Geometry: final body of the model. Coordinates: model frame, mm. A direction names the side the tool comes from. Coordinates: 2 decimals unless noted, no trailing zeros. Order: outer loops, then holes, each group sorted by start corner. A loop starts at its lowest first (then second) coordinate and runs counter-clockwise, first axis right, second up. Notation, with made-up numbers: (33, 87) -> (51, 87) arc R11 cw to (51, 105) -> close; hole circle Ø5 at (73, 64.25). An arc over 180 degrees is marked (long way). Answer in a Markdown table with one row per item. Add a question column.
1) Section query B-B on x = 57.25. Return the cut outline in (y, z).
2) Ray query, line 1 (X direction, y = 0.85, z = -37.25); line 2 (Z direction, x = 46, y = 6.5); line 3 (Y direction, x = 34, z = -15.5). Return the intervals inside material, ascending. Write a range as from..to.
3) Set-up query: faces 5 (the face through (41, 13, -16)), 6 (the face through (20.436, 10, -19)), 7 (the face through (57, 9, -32)). Return all of +Z, -Z, +X, -X, +Y, -Y with unobstructed straight access to the full face (end or side cutting, diameter ignored); none if empty.
4) Contact query for flat-ended pins moving along their axis: P1, Ø2, axis at x = 15.5, z = -25.5, coming from the +Y side; P2, Ø2, axis at y = 6, z = -18, coming from the +X side; P3, Ø8.5, axis at x = 12.5, y = 13, coming from the -Z side. Output: stop coordinate, or through.
5) Section query D-D on x = 13. Return the cut outline in (y, z), then the cut area to 3 significant figures.
6) Pull-direction query (X, two-part tool) for faces 1 (the face through (51, 7, -9.117)), 2 (the face through (2.21, 0.51, -35.96)), 3 (the face through (61.554, 5, -32)), 4 (the face through (52.647, 5, -32)); classes: +X half, -X half, draft (parallel to the pull), parting line (faces both ways), or undercut.
7) Section query A-A on z = -37.25. Return the cut outline in (x, y).
8) Section query C-C on y = 5. Return the cut outline in (x, z), then the cut area to 3 significant figures.
```python
from build123d import *

# Parameters (mm, degrees)
SKETCH1_W           = 60
SKETCH1_H           = 40
BOSS_EXTRUDE1_DEPTH = 1
SKETCH2_R           = 1.4
CUT_EXTRUDE1_DEPTH  = 73.117958928
SKETCH3_R           = 1.794713796
SKETCH3_W           = 11.029321298
SKETCH3_H           = 9.406259618
BOSS_EXTRUDE2_DEPTH = 12
SKETCH4_W           = 8.907146541
SKETCH4_H           = 4.90887134
BOSS_EXTRUDE3_DEPTH = 8
SKETCH5_W           = 7.89622208
SKETCH5_H           = 4.078620146
SKETCH5_W_2         = 8.030698063
BOSS_EXTRUDE4_DEPTH = 18


with BuildPart() as part:
    # Sketch1 → Boss-Extrude1 (new body)
    with BuildSketch(Plane(origin=(0, 0, 0), x_dir=(1, 0, 0), z_dir=(0, 1, 0))):
        with Locations((30, 20)):
            Rectangle(SKETCH1_W, SKETCH1_H)
    extrude(amount=BOSS_EXTRUDE1_DEPTH)

    # Sketch2 → Cut-Extrude1 (cut, through all)
    with BuildSketch(Plane(origin=(0, 1, 0), x_dir=(1, 0, 0), z_dir=(0, 1, 0))):
        with Locations(Location((2.75, 37.25, 0), (0, 0, 270))):
            Circle(SKETCH2_R)
        with Locations(Location((57.25, 37.25, 0), (0, 0, 270))):
            Circle(SKETCH2_R)
        with Locations(Location((57.25, 2.75, 0), (0, 0, 270))):
            Circle(SKETCH2_R)
        with Locations(Location((2.75, 2.75, 0), (0, 0, 270))):
            Circle(SKETCH2_R)
    extrude(amount=-CUT_EXTRUDE1_DEPTH, mode=Mode.SUBTRACT)

    # Sketch3 → Boss-Extrude2 (add)
    with BuildSketch(Plane(origin=(0, 1, 0), x_dir=(1, 0, 0), z_dir=(0, 1, 0))):
        with Locations(Location((41.01670641, 16.304679201, 0), (0, 0, 90))):
            Circle(SKETCH3_R)
        with Locations((50.861034001, 13.82058061)):
            Rectangle(SKETCH3_W, SKETCH3_H)
    extrude(amount=BOSS_EXTRUDE2_DEPTH)

    # Sketch4 → Boss-Extrude3 (add)
    with BuildSketch(Plane(origin=(0, 1, 0), x_dir=(1, 0, 0), z_dir=(0, 1, 0))):
        with Locations((57.100404147, 31.839794384)):
            Rectangle(SKETCH4_W, SKETCH4_H)
    extrude(amount=BOSS_EXTRUDE3_DEPTH)

    # Sketch5 → Boss-Extrude4 (add)
    with BuildSketch(Plane(origin=(0, 1, 0), x_dir=(1, 0, 0), z_dir=(0, 1, 0))):
        with Locations((13.964882377, 18.540826958)):
            Rectangle(SKETCH5_W, SKETCH5_H)
        with Locations((24.451181127, 18.540826958)):
            Rectangle(SKETCH5_W_2, SKETCH5_H)
    extrude(amount=BOSS_EXTRUDE4_DEPTH)


solid = part.part
```
Result:
| question | item | result |
|---|---|---|
| 1 | outline | (0, -40) -> (1, -40) -> (1, -38.65) -> (0, -38.65) -> close; (0, -35.85) -> (1, -35.85) -> (1, -34.29) -> (9, -34.29) -> (9, -29.39) -> (1, -29.39) -> (1, -4.15) -> (0, -4.15) -> close; (0, -1.35) -> (1, -1.35) -> (1, 0) -> (0, 0) -> close |
| 2 | line 1 | 0..1.35, 4.15..55.85, 58.65..60 |
| 2 | line 2 | -18.52..-9.12 |
| 2 | line 3 | 0..1 |
| 3 | face 5 | +Z, -Z, +X, +Y |
| 3 | face 6 | +Z, -Z, +Y |
| 3 | face 7 | -Z, +X, -X, +Y |
| 4 | P1 | y = 1 |
| 4 | P2 | x = 56.38 |
| 4 | P3 | z = -20.58 |
| 5 | outline | (0, -40) -> (1, -40) -> (1, -20.58) -> (19, -20.58) -> (19, -16.5) -> (1, -16.5) -> (1, 0) -> (0, 0) -> close |
| 5 | area | 113 mm2 |
| 6 | face 1 | draft |
| 6 | face 2 | undercut |
| 6 | face 3 | +X half |
| 6 | face 4 | -X half |
| 7 | outline | (0, 0) -> (1.35, 0) -> (1.35, 1) -> (0, 1) -> close; (4.15, 0) -> (55.85, 0) -> (55.85, 1) -> (4.15, 1) -> close; (58.65, 0) -> (60, 0) -> (60, 1) -> (58.65, 1) -> close |
| 8 | outline | (10.02, -20.58) -> (17.91, -20.58) -> (17.91, -16.5) -> (10.02, -16.5) -> close; (20.44, -20.58) -> (28.47, -20.58) -> (28.47, -16.5) -> (20.44, -16.5) -> close; circle Ø3.59 at (41.02, -16.3); (45.35, -18.52) -> (56.38, -18.52) -> (56.38, -9.12) -> (45.35, -9.12) -> close; (52.65, -34.29) -> (61.55, -34.29) -> (61.55, -29.39) -> (52.65, -29.39) -> close |
| 8 | area | 223 mm2 |
